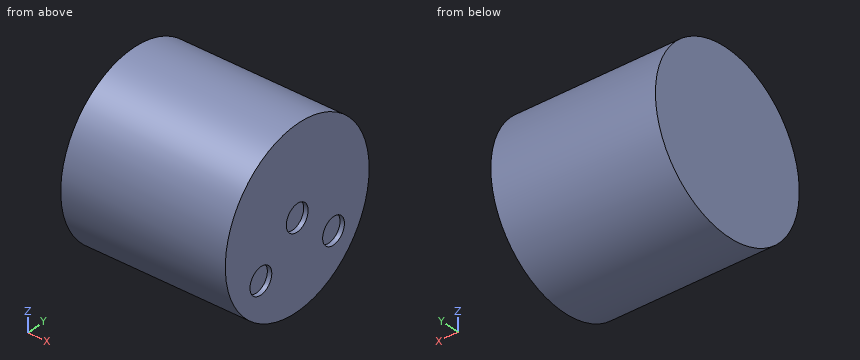
Autodesk Inventor part; units mm, degrees
ref_plane "YZ Plane" through (0, 0, 0) normal (1, 0, 0) x (0, 1, 0)
ref_plane "XZ Plane" through (0, 0, 0) normal (0, 1, 0) x (-1, 0, 0)
ref_plane "XY Plane" through (0, 0, 0) normal (0, 0, 1) x (1, 0, 0)
sketch "スケッチ1" plane through (0, 0, 0) normal (0, 0, 1) x (1, 0, 0)
  point P0 (0, 0)
sketch "スケッチ2" plane through (0, 0, 0) normal (1, 0, 0) x (0, 1, 0)
  circle A0 centre (0, 0) radius 9.9
  dimension "d0" = 19.8
extrude "押し出し1" add sketch "スケッチ2" along normal blind 18.5
sketch "スケッチ3" plane through (18.5, 0, 0) normal (1, 0, 0) x (0, 0, -1)
  circle A0 centre (0, 0) radius 1.5
  dimension "d3" = 3
extrude "押し出し2" cut sketch "スケッチ3" against normal blind 0.5
sketch "スケッチ4" plane through (18.5, 0, 0) normal (1, 0, 0) x (0, 0, -1)
  circle A0 centre (4, 5) radius 1.5
  circle A1 centre (4, -5) radius 1.5
  point P0 (0, 0)
  dimension "d6" = 3
  dimension "d7" = 3
extrude "押し出し3" cut sketch "スケッチ4" against normal blind 0.5
properties part number "stepping_motor" material "アルミニウム"
Can you work these out from the model? Positions are in its coordinate system, mm. Coordinates: 2 decimals unless noted, no trailing zeros. Loops run counter-clockwise (first coordinate to the right, second up) from the corner with the lowest first, then second, coordinate; pieces in that order, holes last. Notation, with made-up numbers: (31, -17) - (70, -17) arc R17 ccw to (70, 0) - close; hole circle Ø3 at (-7, -38.75). An arc over 180 degrees is marked (long way). Put each result on its own line as item: value. Start each with the question number.
Item 1: Suppose I cut it at A-A (y = 5). Please give me the cut outline in (x, z).
Item 2: Suppose I cut it at D-D (y = -6). Please give me the cut outline in (x, z).
Item 3: Suppose I cut it at C-C (x = 11.5). Please give me the cut outline in (y, z), and give its area (3 significant figures).
Item 4: For pin 1 (2 mm diameter, centred on x = 15, y = -5, fed in from +Z); pin 2 (2.5 mm diameter, centred on y = 0, z = 0, fed in from +X); pin 3 (4 mm diameter, centred on x = 4.5, y = 5, fed in from -Z), each with a flat end and sliding along its axis, tell me the tip position at first contact or that it passes through.
Item 5: Suppose I cut it at B-B (z = -5). Please give me the cut outline in (x, y), and give its area (3 significant figures).
Item 6: If I drill on line 1 along Y through (x, z) = (18.15, -4); line 2 along Z through (x, y) = (7.5, -9); line 3 along Z through (x, y) = (3.5, 6.25), over which ranges is the centre line in solid material (lowest first)?
Here are the results:
1. outline: (0, -8.54) - (18.5, -8.54) - (18.5, -5.5) - (18, -5.5) - (18, -2.5) - (18.5, -2.5) - (18.5, 8.54) - (0, 8.54) - close
2. outline: (0, -7.87) - (18.5, -7.87) - (18.5, -5.12) - (18, -5.12) - (18, -2.88) - (18.5, -2.88) - (18.5, 7.87) - (0, 7.87) - close
3. outline: circle Ø19.8 at (0, 0)
3. area: 308 mm²
4. pin 1: z = 9.06
4. pin 2: x = 18
4. pin 3: z = -9.43
5. outline: (0, -8.54) - (18.5, -8.54) - (18.5, -6.12) - (18, -6.12) - (18, -3.88) - (18.5, -3.88) - (18.5, 3.88) - (18, 3.88) - (18, 6.12) - (18.5, 6.12) - (18.5, 8.54) - (0, 8.54) - close
5. area: 314 mm²
6. line 1: -9.06 to -6.5, -3.5 to 3.5, 6.5 to 9.06
6. line 2: -4.12 to 4.12
6. line 3: -7.68 to 7.68
